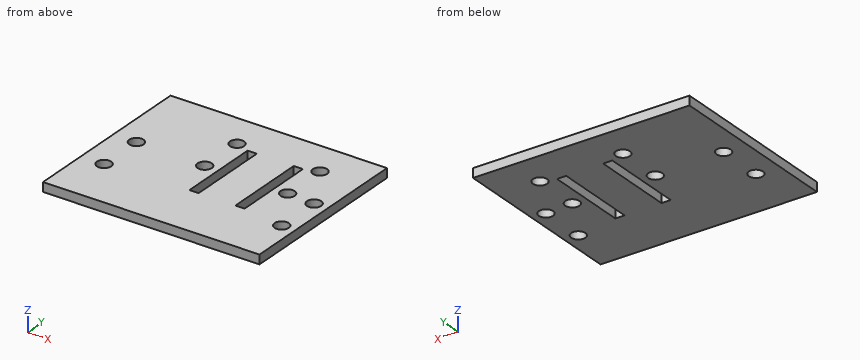
```python
from build123d import *

# Parameters (mm, degrees)
SKETCH_1_W      = 47
SKETCH_1_H      = 39.4
SKETCH_1_R      = 1.55
SKETCH_1_W_2    = 2
SKETCH_1_H_2    = 18
EXTRUDE_1_DEPTH = 2


with BuildPart() as part:
    # 草图1 → 凸台-拉伸1 (new body)
    with BuildSketch(Plane.XY):
        Rectangle(SKETCH_1_W, SKETCH_1_H)
        with Locations((20.5, 1.43)):
            Circle(SKETCH_1_R, mode=Mode.SUBTRACT)
        with Locations((20.5, -8.57)):
            Circle(SKETCH_1_R, mode=Mode.SUBTRACT)
        with Locations((-18.5, 2.05)):
            Circle(SKETCH_1_R, mode=Mode.SUBTRACT)
        with Locations((-18.5, -7.95)):
            Circle(SKETCH_1_R, mode=Mode.SUBTRACT)
        with Locations((-3.499999601, 11.8)):
            Circle(SKETCH_1_R, mode=Mode.SUBTRACT)
        with Locations((-3.5, 1.8)):
            Circle(SKETCH_1_R, mode=Mode.SUBTRACT)
        with Locations((14.5, 11.8)):
            Circle(SKETCH_1_R, mode=Mode.SUBTRACT)
        with Locations((14.5, 1.8)):
            Circle(SKETCH_1_R, mode=Mode.SUBTRACT)
        with Locations((10.5, 1.8)):
            Rectangle(SKETCH_1_W_2, SKETCH_1_H_2, mode=Mode.SUBTRACT)
        with Locations((0.5, 1.8)):
            Rectangle(SKETCH_1_W_2, SKETCH_1_H_2, mode=Mode.SUBTRACT)
    extrude(amount=EXTRUDE_1_DEPTH)


solid = part.part
```
CAD build for the part. Positions are in the model's coordinates, mm. Round coordinates to 2 decimals unless told otherwise and drop trailing zeros. Write each loop counter-clockwise with the first axis right and the second up, starting at its lowest first coordinate (ties: lowest second). Pieces come first, ordered by that corner, then holes. Notation, with made-up numbers: (61, -14) - (75, -14) arc R23 ccw to (75, -3) - close; hole circle Ø7 at (19.5, 67). An arc over 180 degrees is marked (long way). Write item = value, one per line. Start each with the question number.
Q1. Band-saw the part on A-A (x = -3.5). Give the cut face in (y, z), then the cut area to 3 significant figures.
Q2. Drop flat-ended pins along their axis: pin 1 (1.9 mm diameter, centred on x = -3.5, y = 1.8, fed in from -Z); pin 2 (3.5 mm diameter, centred on x = 20.5, y = 1.43, fed in from -Z). Give the stop position or say it passes through.
Q3. Band-saw the part on B-B (y = -8.57). Give the cut face in (x, z), then the cut area to 3 significant figures.
Q4. Band-saw the part on C-C (z = 0.3). Count the separate pieces of the cut face and the enclosed holes in it, then the cut area to 3 significant figures.
Q5. Probe L1, parallel to X at y = -3.5, z = 1.15; L2, parallel to Y at x = 14.5, z = 1.45; L3, parallel to Y at x = 20.5, z = 1.2. List the from-to ranges inside material, lowest first. Write a range as from..to.
Answers below:
q1.outline = (-19.7, 0) - (0.25, 0) - (0.25, 2) - (-19.7, 2) - close; (3.35, 0) - (10.25, 0) - (10.25, 2) - (3.35, 2) - close; (13.35, 0) - (19.7, 0) - (19.7, 2) - (13.35, 2) - close
q1.area = 66.4 mm2
q2.pin_1 = through
q2.pin_2 = 0
q3.outline = (-23.5, 0) - (-19.92, 0) - (-19.92, 2) - (-23.5, 2) - close; (-17.08, 0) - (18.95, 0) - (18.95, 2) - (-17.08, 2) - close; (22.05, 0) - (23.5, 0) - (23.5, 2) - (22.05, 2) - close
q3.area = 82.1 mm2
q4.separate_pieces = 1
q4.enclosed_holes = 10
q4.area = 1,720 mm2
q5.L1 = -23.5..-0.5, 1.5..9.5, 11.5..23.5
q5.L2 = -19.7..0.25, 3.35..10.25, 13.35..19.7
q5.L3 = -19.7..-10.12, -7.02..-0.12, 2.98..19.7
